Geometry check sheet. Reference: the model listing, model coordinates, mm. A direction names the side the tool comes from. Round coordinates to 2 decimals unless told otherwise and drop trailing zeros. Loops run counter-clockwise (first coordinate to the right, second up) from the corner with the lowest first, then second, coordinate; pieces in that order, holes last. Notation, with made-up numbers: M -17.5,-14 L 31.5,-14 A24 ccw 31.5,-1 Z; hole C 81.25,31 d3. An arc over 180 degrees is marked long. Write item = value, one per line.
from build123d import *

# Parameters (mm, degrees)
SKETCH1_W               = 1187.5
SKETCH1_H               = 950
SKETCH1_W_2             = 1000
SKETCH1_H_2             = 800
BOSS_EXTRUDE1_DEPTH     = 50
SKETCH2_W               = 93.75
SKETCH2_H               = 75
BOSS_EXTRUDE2_DEPTH     = 800
SKETCH3_W               = 950
SKETCH3_H               = 75
BOSS_EXTRUDE3_DEPTH     = 93.75
SKETCH4_W               = 950
SKETCH4_H               = 75
BOSS_EXTRUDE4_DEPTH     = 93.75
CUT_EXTRUDE1_DEPTH      = 2000
CUT_EXTRUDE1_DEPTH_BACK = 2000
SKETCH5_R               = 27.5


with BuildPart() as part:
    # Sketch1 → Boss-Extrude1 (new body)
    with BuildSketch(Plane(origin=(0, 0, 0), x_dir=(1, 0, 0), z_dir=(0, 1, 0))):
        Rectangle(SKETCH1_W, SKETCH1_H)
        Rectangle(SKETCH1_W_2, SKETCH1_H_2, mode=Mode.SUBTRACT)
    boss_extrude1 = extrude(amount=BOSS_EXTRUDE1_DEPTH)

    # Sketch2 → Boss-Extrude2 (add)
    with BuildSketch(Plane(origin=(0, 50, 0), x_dir=(1, 0, 0), z_dir=(0, 1, 0))):
        with Locations((-546.875, 437.5)):
            Rectangle(SKETCH2_W, SKETCH2_H)
        with Locations((-546.875, -437.5)):
            Rectangle(SKETCH2_W, SKETCH2_H)
        with Locations((546.875, 437.5)):
            Rectangle(SKETCH2_W, SKETCH2_H)
        with Locations((546.875, -437.5)):
            Rectangle(SKETCH2_W, SKETCH2_H)
    extrude(amount=BOSS_EXTRUDE2_DEPTH)

    # Mirror1: Boss-Extrude1 across plane
    add(boss_extrude1.mirror(Plane.ZX.offset(450)))

    # Sketch3 → Boss-Extrude3 (add)
    with BuildSketch(Plane(origin=(593.75, 0, 0), x_dir=(0, 0, -1), z_dir=(1, 0, 0))):
        with Locations((0, 450)):
            Rectangle(SKETCH3_W, SKETCH3_H)
    extrude(amount=-BOSS_EXTRUDE3_DEPTH)

    # Sketch4 → Boss-Extrude4 (add)
    with BuildSketch(Plane.ZY.offset(593.75)):
        with Locations((0, 450)):
            Rectangle(SKETCH4_W, SKETCH4_H)
    extrude(amount=-BOSS_EXTRUDE4_DEPTH)

    # Sketch5 → Cut-Extrude1 (cut, two sides: drawn at the far end of the back side and taken through both)
    with BuildSketch(Plane(origin=(593.75, 0, 0), x_dir=(0, 0, -1), z_dir=(1, 0, 0)).offset(-CUT_EXTRUDE1_DEPTH_BACK)):
        with Locations(Location((0, 450, 0), (0, 0, 180))):
            Circle(SKETCH5_R)
    extrude(amount=CUT_EXTRUDE1_DEPTH + CUT_EXTRUDE1_DEPTH_BACK, mode=Mode.SUBTRACT)


solid = part.part
(1) Sectioned sample at B-B on y = 777.5. Record the cut outline in (x, z), then the cut area to 3 significant figures.
Result set:
outline = M -593.75,-475 L -500,-475 L -500,-400 L -593.75,-400 Z; M -593.75,400 L -500,400 L -500,475 L -593.75,475 Z; M 500,-475 L 593.75,-475 L 593.75,-400 L 500,-400 Z; M 500,400 L 593.75,400 L 593.75,475 L 500,475 Z
area = 28,100 mm2
(2) Sectioned sample at C-C on x = 153. Record the cut outline in (y, z), then the cut area to 3 significant figures.
Result set:
outline = M 0,-475 L 50,-475 L 50,-400 L 0,-400 Z; M 0,400 L 50,400 L 50,475 L 0,475 Z; M 850,-475 L 900,-475 L 900,-400 L 850,-400 Z; M 850,400 L 900,400 L 900,475 L 850,475 Z
area = 15,000 mm2
(3) Sectioned sample at A-A on z = 77. Record the cut outline in (x, y), then the cut area to 3 significant figures.
Result set:
outline = M -593.75,0 L -500,0 L -500,50 L -593.75,50 Z; M -593.75,412.5 L -500,412.5 L -500,487.5 L -593.75,487.5 Z; M -593.75,850 L -500,850 L -500,900 L -593.75,900 Z; M 500,0 L 593.75,0 L 593.75,50 L 500,50 Z; M 500,412.5 L 593.75,412.5 L 593.75,487.5 L 500,487.5 Z; M 500,850 L 593.75,850 L 593.75,900 L 500,900 Z
area = 32,800 mm2
(4) Release check for a two-part mould opening along X. For faces 1 (the flat face through (546, 850, -6)), 2 (the flat face through (593.75, 456, 112)), 3 (the flat face through (-7, 25, -400)), 4 (the flat face through (-593.75, 456, 112)) record: released by +X, released by -X, zero draft, split by the parting line, or undercut.
Result set:
face_1 = zero draft
face_2 = released by +X
face_3 = undercut
face_4 = released by -X
(5) Material ranges on line 1 along Y through (x, z) = (523, 0); line 2 along X through (y, z) = (459, 33); line 3 along Z through (x, y) = (520.5, 461), recorded low to high. Write a range as from..to.
Result set:
line_1 = 0..50, 412.5..422.5, 477.5..487.5, 850..900
line_2 = -593.75..-500, 500..593.75
line_3 = -475..-25.2, 25.2..475
(6) Tool access check on faces 5 (the flat face through (-8, 0, 416)), 6 (the flat face through (500, 419, 2)), 7 (the flat face through (-548, 487.5, -6)), 8 (the flat face through (-500, 25, 6)). Record the directions out of +Z, -Z, +X, -X, +Y, -Y that give a thin tool (end or side, any length) a straight path to the whole face; none if there is none.
Result set:
face_5 = +Z, -Z, +X, -X, -Y
face_6 = +Z, -Z
face_7 = +X, -X
face_8 = +Y, -Y
